Build history of the part. All positions in model axes, mm. Face numbers are marked on the shaded views. Round coordinates to 2 decimals unless told otherwise and drop trailing zeros. Write each loop counter-clockwise with the first axis right and the second up, starting at its lowest first coordinate (ties: lowest second). Pieces come first, ordered by that corner, then holes. Notation, with made-up numbers: (6, 32) - (26, 32) arc R31 ccw to (26, 57) - close; hole circle Ø10 at (-19.5, 72.5). An arc over 180 degrees is marked (long way). Answer as a JSON object with one key per item and string values. Group by question number.
Item 1: Slice it at B-B, the plane x = 2.85. List the corners of the cut face in (y, z).
Item 2: Two-plate mould, pull along X, no slides. Class the marked faces 1, 2, 3 and 4: +X half, -X half, draft (parallel to the pull), parting line (faces both ways), or undercut.
Item 3: Slice it at C-C, the plane z = 1.7. List the corners of the cut face in (x, y).
Item 4: Probe line 1 (Y direction, x = 20.15, z = 1.4); line 2 (X direction, y = 15.25, z = 1.55); line 3 (X direction, y = 16, z = 0.8). List the from-to ranges inside material, lowest first. Write a range as from..to.
Item 5: Flat gauge pin, fed straight in: pin 1 (4 mm diameter, centred on x = 20.15, y = 2.25, fed in from +Z). Where does the tip first touch, or does it go through?
Item 6: Slice it at A-A, the plane y = 15.25. List the corners of the cut face in (x, z), then the cut area to 3 significant figures.
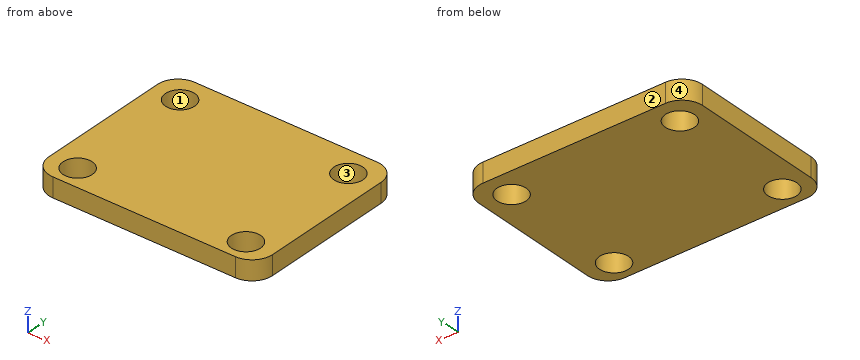
from build123d import *

# Parameters (mm, degrees)
PAD_DEPTH    = 2
SKETCH001_R  = 1.5
POCKET_DEPTH = 2.001


with BuildPart() as part:
    # Sketch → Pad (new body)
    with BuildSketch(Plane.XY):
        with BuildLine():
            Line((0, 15.87868), (0, 2.12132))
            ThreePointArc((0, 2.12132), (0.62132, 0.62132), (2.12132, 0))
            Line((2.12132, 0), (20.87868, 0))
            ThreePointArc((20.87868, 0), (22.37868, 0.62132), (23, 2.12132))
            Line((23, 2.12132), (23, 15.87868))
            ThreePointArc((23, 15.87868), (22.37868, 17.37868), (20.87868, 18))
            Line((20.87868, 18), (2.12132, 18))
            ThreePointArc((2.12132, 18), (0.62132, 17.37868), (0, 15.87868))
        make_face()
    extrude(amount=PAD_DEPTH)

    # Sketch001 → Pocket (cut, through all)
    with BuildSketch(Plane.XY):
        with Locations((20.15, 15.25)):
            Circle(SKETCH001_R)
        with Locations((2.85, 15.25)):
            Circle(SKETCH001_R)
        with Locations((2.85, 2.25)):
            Circle(SKETCH001_R)
        with Locations((20.15, 2.25)):
            Circle(SKETCH001_R)
    extrude(amount=POCKET_DEPTH, mode=Mode.SUBTRACT)


solid = part.part
Geometry says:
{
 "1": {"outline": "(0, 0) - (0.75, 0) - (0.75, 2) - (0, 2) - close; (3.75, 0) - (13.75, 0) - (13.75, 2) - (3.75, 2) - close; (16.75, 0) - (18, 0) - (18, 2) - (16.75, 2) - close"},
 "2": {"face 1": "undercut", "face 2": "draft", "face 3": "undercut", "face 4": "-X half"},
 "3": {"outline": "(0, 2.12) arc R2.12 ccw to (2.12, 0) - (20.88, 0) arc R2.12 ccw to (23, 2.12) - (23, 15.88) arc R2.12 ccw to (20.88, 18) - (2.12, 18) arc R2.12 ccw to (0, 15.88) - close; hole circle Ø3 at (2.85, 2.25); hole circle Ø3 at (2.85, 15.25); hole circle Ø3 at (20.15, 2.25); hole circle Ø3 at (20.15, 15.25)"},
 "4": {"line 1": "y = 0..0.75, 3.75..13.75, 16.75..18", "line 2": "x = 0..1.35, 4.35..18.65, 21.65..23", "line 3": "x = 0..1.55, 4.15..18.85, 21.45..23"},
 "5": {"pin 1": "stops at z = 2"},
 "6": {"outline": "(0, 0) - (1.35, 0) - (1.35, 2) - (0, 2) - close; (4.35, 0) - (18.65, 0) - (18.65, 2) - (4.35, 2) - close; (21.65, 0) - (23, 0) - (23, 2) - (21.65, 2) - close", "area": "34.0 mm^2"}
}
